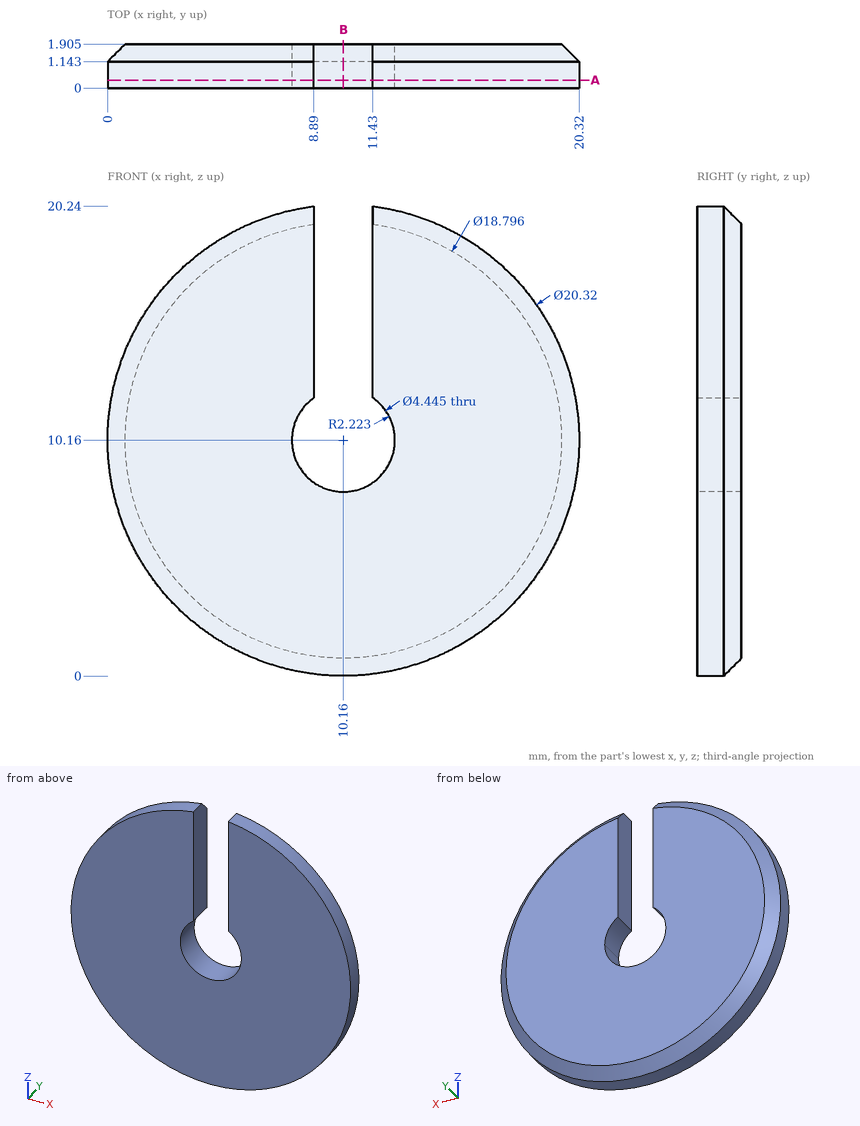
Can you work these out from the drawing? Everything is in mm from the part's minimum corner. Round coordinates to 2 decimals unless told otherwise and drop trailing zeros. Order: outer loops, then holes, each group sorted by start corner. A loop starts at its lowest first (then second) coordinate and runs counter-clockwise, first axis right, second up. Notation, with made-up numbers: (-29.5, 72.5) -> (4.5, 72.5) arc R10 cw to (4.5, 86.5) -> close; hole circle Ø3 at (65, -8). An arc over 180 degrees is marked (long way). Use CSV: the item, a comma, the result in double quotes.
1. I want a section at A-A on y = 0.35. List the corners of the cut face in (x, z) for me (1 decimal), and give its area (3 significant figures).
Recorded:
outline,"(8.9, 12) -> (8.9, 20.2) arc R10.2 ccw (long way) to (11.4, 20.2) -> (11.4, 12) arc R2.2 cw (long way) to start"
area,"288 mm2"
2. I want a section at B-B on x = 10.16. List the corners of the cut face in (y, z) for me (1 decimal), and give its area (3 significant figures).
Recorded:
outline,"(0, 0) -> (1.1, 0) -> (1.9, 0.8) -> (1.9, 7.9) -> (0, 7.9) -> close"
area,"14.8 mm2"
3. I'm going to push flat-ended pins straight in: P1, Ø1, axis at y = 1.5, z = 6, coming from the -X side; P2, Ø1, axis at x = 12.5, y = 1.5, coming from the +Z side. Where does each tip first touch, or does it pass through?
Recorded:
P1,"stops at x = 0.74"
P2,"stops at z = 20.12"
4. I need wall thicknesses on line 1 along Z through (x, y) = (10.16, 0.45); line 2 along X through (y, z) = (1.5, 10.16) (1 decimal); line 3 along X through (y, z) = (1.4, 10.16) (1 decimal). Which ranges of each line are inside material? Lowest first, please.
Recorded:
line 1,"z = 0 to 7.94"
line 2,"x = 0.4 to 7.9, 12.4 to 20"
line 3,"x = 0.3 to 7.9, 12.4 to 20.1"
